Autodesk Inventor part; units mm, degrees
ref_plane "YZ Plane" through (0, 0, 0) normal (1, 0, 0) x (0, 1, 0)
ref_plane "XZ Plane" through (0, 0, 0) normal (0, 1, 0) x (-1, 0, 0)
ref_plane "XY Plane" through (0, 0, 0) normal (0, 0, 1) x (1, 0, 0)
sketch "Sketch1" plane through (0, 0, 0) normal (0, 1, 0) x (-1, 0, 0)
  line L0 (4.175, 0) -> (36.175, 0)
  line L1 (40.35, 4.175) -> (40.35, 36.175)
  line L2 (36.175, 40.35) -> (4.175, 40.35)
  line L3 (0, 36.175) -> (0, 4.175)
  circle A0 centre (4.175, 4.175) radius 1.5
  circle A1 centre (36.175, 4.175) radius 1.5
  circle A2 centre (4.175, 36.175) radius 1.5
  circle A3 centre (36.175, 36.175) radius 1.5
  arc A4 (4.175, 40.35) -> (0, 36.175) centre (4.175, 36.175) ccw
  arc A5 (40.35, 36.175) -> (36.175, 40.35) centre (36.175, 36.175) ccw
  arc A6 (36.175, 0) -> (40.35, 4.175) centre (36.175, 4.175) ccw
  arc A7 (0, 4.175) -> (4.175, 0) centre (4.175, 4.175) ccw
  circle A8 centre (20.175, 20.175) radius 19
  point P0 (0, 0)
  point P1 (40.35, 0)
  point P2 (40.35, 40.35)
  dimension "d0" = 40.35
  dimension "d1" = 40.35
  dimension "d2" = 3
  dimension "d5" = 32
  dimension "d8" = 32
  dimension "d12" = 4.175
  dimension "d15" = 38
  dimension "d16" = 20.175
  dimension "d17" = 20.175
extrude "Extrusion2" add sketch "Sketch1" along normal blind 10
properties part number "Ventilador" material "Rubber, Silicone"
Design review of the part built by this model. Coordinates are the model's own, in mm. Coordinates: 2 decimals unless noted, no trailing zeros. Loops run counter-clockwise (first coordinate to the right, second up) from the corner with the lowest first, then second, coordinate; pieces in that order, holes last. Notation, with made-up numbers: M 81.5,72.25 L 106.5,72.25 A9 cw 106.5,88.25 Z; hole C 4,12.5 d1. An arc over 180 degrees is marked long. One line per question, with ' | ' between items.
(1) We need section C-C (y = 5.5). Give the boundary of the cut face in (x, z) (3 decimals), and give its area (3 significant figures).
Filled in:
outline: M -40.35,4.175 A4.175 ccw -36.175,0 L -4.175,0 A4.175 ccw 0,4.175 L 0,36.175 A4.175 ccw -4.175,40.35 L -36.175,40.35 A4.175 ccw -40.35,36.175 Z; hole C -20.175,20.175 d38; hole C -36.175,4.175 d3; hole C -36.175,36.175 d3; hole C -4.175,4.175 d3; hole C -4.175,36.175 d3 | area: 451 mm^2
(2) We need section B-B (x = -25). Give the boundary of the cut face in (y, z), and give its area (3 significant figures).
Filled in:
outline: M 0,0 L 10,0 L 10,1.8 L 0,1.8 Z; M 0,38.55 L 10,38.55 L 10,40.35 L 0,40.35 Z | area: 36.0 mm^2
(3) We need section A-A (z = 31). Give the boundary of the cut face in (x, y).
Filled in:
outline: M -40.35,0 L -35.79,0 L -35.79,10 L -40.35,10 Z; M -4.56,0 L 0,0 L 0,10 L -4.56,10 Z
(4) Wall thickness on probe 1 along Z at (x, y) = (-20.5, 8.5); probe 2 along Z at (x, y) = (-35.5, 8.5); probe 3 along Z at (x, y) = (-3.5, 7): over which ranges is each line inside the solid? List them lowest first.
Filled in:
probe 1: z = 0 to 1.18, 39.17 to 40.35 | probe 2: z = 0 to 2.84, 5.51 to 8.94, 31.41 to 34.84, 37.51 to 40.35 | probe 3: z = 0.05 to 2.84, 5.51 to 11.07, 29.28 to 34.84, 37.51 to 40.3
(5) For pin 1 Ø1.8 at (x, z) = (-4.175, 36.175) entering from -Y, flat-tipped, find the tip position at first contact; note if it passes through.
Filled in:
pin 1: passes through
(6) We need section D-D (z = 3.5). Give the boundary of the cut face in (x, y).
Filled in:
outline: M -40.3,0 L -37.51,0 L -37.51,10 L -40.3,10 Z; M -34.84,0 L -29.28,0 L -29.28,10 L -34.84,10 Z; M -11.07,0 L -5.51,0 L -5.51,10 L -11.07,10 Z; M -2.84,0 L -0.05,0 L -0.05,10 L -2.84,10 Z
(7) Draft analysis for pull direction Z (two halves, no side actions). For faces 1 (the face through (-3.98, 4.93, 34.688)), 2 (the face through (-1.255, 4.93, 1.191)), 3 (the face through (-40.35, 5, 20)), state which applies: released by +Z, released by -Z, zero draft, split by the parting line, or undercut.
Filled in:
face 1: undercut | face 2: released by -Z | face 3: zero draft
